Design review of the part built by this model. Coordinates are the model's own, in mm. Round coordinates to 2 decimals unless told otherwise and drop trailing zeros. Loops run counter-clockwise (first coordinate to the right, second up) from the corner with the lowest first, then second, coordinate; pieces in that order, holes last. Notation, with made-up numbers: (56, -13) - (61, -13) arc R16 cw to (61, 0) - close; hole circle Ø1 at (79.5, 44.25). An arc over 180 degrees is marked (long way). Return JSON: item names as keys, results as strings. Group by question number.
(1) We need section C-C, the plane x = 0.5. Write out the cut boundary in (y, z), and give its area (3 significant figures).
(2) We need section D-D, the plane z = -4. Write out the cut boundary in (x, y), and give its area (3 significant figures).
(3) Wall thickness on L1, parallel to X at y = 1.15, z = -4.5; L2, parallel to Y at x = 0.2, z = 1.75; L3, parallel to Z at x = 0.1, y = -1.1: over which ranges is each line inside the solid? List them lowest first. Write a range as [from, to].
(4) We need section A-A, the plane z = 0. Write out the cut boundary in (x, y), and give its area (3 significant figures).
Autodesk Inventor part; units mm, degrees
ref_plane "Plano de trabajo1" through (0, 0, -1.3) normal (0, 0, 1) x (1, 0, 0)
ref_plane "YZ Plane" through (0, 0, 0) normal (1, 0, 0) x (0, 1, 0)
ref_plane "XZ Plane" through (0, 0, 0) normal (0, 1, 0) x (-1, 0, 0)
sketch "Boceto1" plane through (0, 0, 0) normal (1, 0, 0) x (0, 1, 0)
  circle A0 centre (0, 0) radius 2.15
  dimension "d0" = 4.3
extrude "Extrusión1" add sketch "Boceto1" along normal mid plane 1.2
fillet "Empalme1" radius 0.5 1 edges at (0.6, -2.15, 0)
fillet "Empalme2" radius 0.5 1 edges at (-0.6, -2.15, 0)
sketch "Boceto2" plane through (-0.6, 0, 0) normal (-1, 0, 0) x (0, 0, 1)
  line L0 (-0.4973, -1.1141) -> (-0.471, 1.1369) construction
  line L1 (-0.471, 1.1369) -> (0.5703, 1.1247) construction
  line L2 (0.5703, 1.1247) -> (0.544, -1.1263) construction
  line L3 (0.544, -1.1263) -> (-0.4973, -1.1141) construction
  line L4 (-0.4973, -1.1141) -> (-0.471, 1.1369) construction
  line L5 (-0.471, 1.1369) -> (0.5703, 1.1247) construction
  line L6 (0.5703, 1.1247) -> (0.544, -1.1263) construction
  line L7 (0.544, -1.1263) -> (-0.4973, -1.1141) construction
  line L8 (-0.4973, -1.1141) -> (-0.471, 1.1369) construction
  line L9 (-0.471, 1.1369) -> (0.5703, 1.1247) construction
  line L10 (0.5703, 1.1247) -> (0.544, -1.1263) construction
  line L11 (0.544, -1.1263) -> (-0.4973, -1.1141) construction
  line L12 (-0.4973, -1.1141) -> (-0.471, 1.1369) construction
  line L13 (-0.471, 1.1369) -> (0.5703, 1.1247) construction
  line L14 (0.5703, 1.1247) -> (0.544, -1.1263) construction
  line L15 (0.544, -1.1263) -> (-0.4973, -1.1141) construction
  line L16 (0.5613, 1.1178) -> (0.5386, -1.1333) construction
  line L17 (0.5386, -1.1333) -> (-0.5027, -1.1227) construction
  line L18 (-0.5027, -1.1227) -> (-0.4799, 1.1284) construction
  line L19 (-0.4799, 1.1284) -> (0.5613, 1.1178) construction
  point P0 (0, 0)
sketch "Boceto3" plane through (0.6, 0, 0) normal (1, 0, 0) x (0, 0, -1)
  line L0 (-0.4973, -1.1141) -> (-0.471, 1.1369) construction
  line L1 (-0.471, 1.1369) -> (0.5703, 1.1247) construction
  line L2 (0.5703, 1.1247) -> (0.544, -1.1263) construction
  line L3 (0.544, -1.1263) -> (-0.4973, -1.1141) construction
  point P0 (0, 0)
ref_plane "Plano de trabajo1" through (0, 0, -1.3) normal (0, 0, 1) x (1, 0, 0)
sketch "Boceto4" plane through (0, 0, -1.3) normal (0, 0, 1) x (1, 0, 0)
  line L0 (0.1, -2.15) -> (0.1, 2.15)
  line L1 (0.6, 1.65) -> (0.6, -1.65)
  line L2 (-0.1, 2.15) -> (-0.1, -2.15)
  line L3 (-0.6, -1.65) -> (-0.6, 1.65)
  line L4 (0.1, -2.15) -> (0.1, 2.15)
  line L5 (-0.1, 2.15) -> (-0.1, -2.15)
  circle A0 centre (0, -1.0922) radius 0.15
  circle A1 centre (0, 1.152) radius 0.15
  point P0 (0, 0)
  dimension "d7" = 0.3
  dimension "d8" = 0.3
extrude "Extrusión2" add sketch "Boceto4" against normal blind 4 contours A0 L2 L0 | L0 A0 | A0 L2 | A1 L2 L0 | L0 A1 | A1 L2
properties part number "cap334"
Solutions:
{
 "1": {"outline": "circle Ø3.9 at (0, 0)", "area": "11.9 mm^2"},
 "2": {"outline": "circle Ø0.3 at (0, -1.09); circle Ø0.3 at (0, 1.15)", "area": "0.141 mm^2"},
 "3": {"L1": "[-0.15, 0.15]", "L2": "[-1.23, 1.23]", "L3": "[-5.3, 1.85]"},
 "4": {"outline": "(-0.6, -1.65) arc R0.5 ccw to (-0.1, -2.15) - (0.1, -2.15) arc R0.5 ccw to (0.6, -1.65) - (0.6, 1.65) arc R0.5 ccw to (0.1, 2.15) - (-0.1, 2.15) arc R0.5 ccw to (-0.6, 1.65) - close", "area": "4.95 mm^2"}
}
